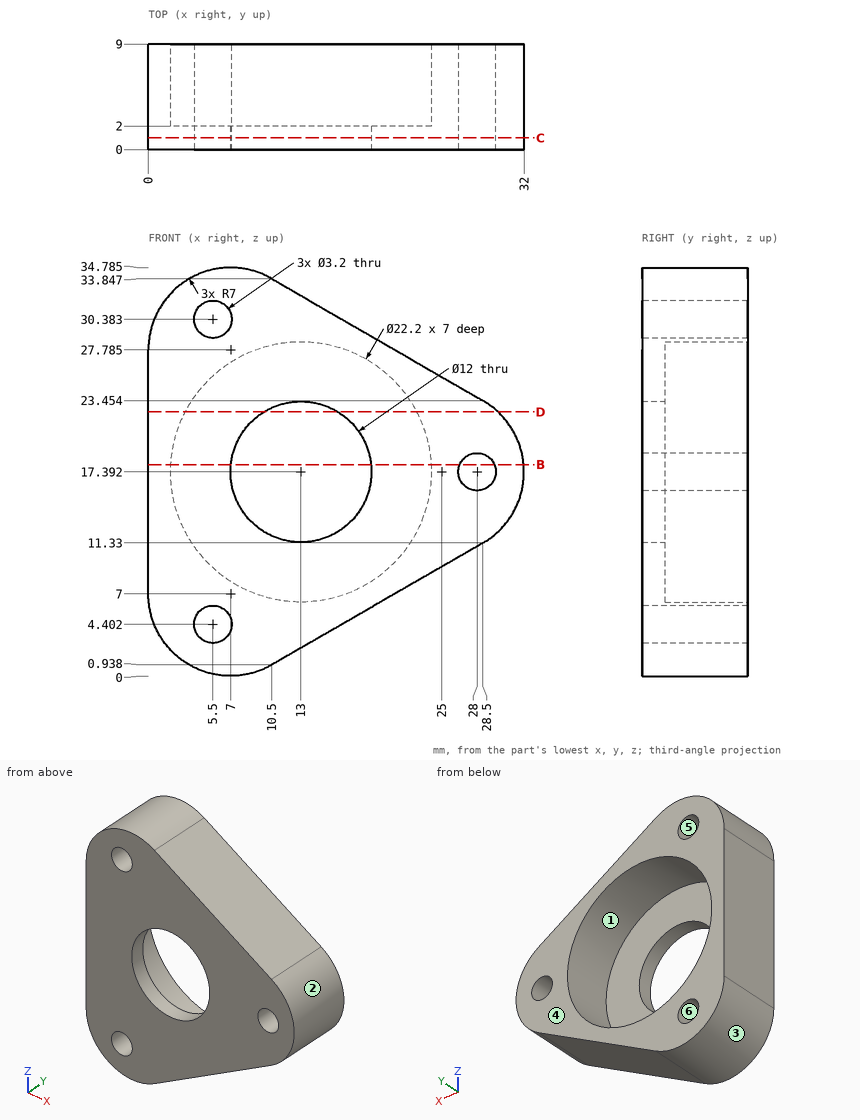
Here's the drawing with two shaded views (mm, measured from the low corner). I have some questions. A direction names the side the tool comes from. Coordinates: 2 decimals unless noted, no trailing zeros. Loops run counter-clockwise (first coordinate to the right, second up) from the corner with the lowest first, then second, coordinate; pieces in that order, holes last.
Item 1: Suppose I cut it at C-C (y = 1). Please give me the cut outline in (x, z) (1 decimal), then the cut area to 3 significant figures.
Answers below:
outline: (0, 7) arc R7 ccw to (10.5, 0.9) - (28.5, 11.3) arc R7 ccw to (28.5, 23.5) - (10.5, 33.8) arc R7 ccw to (0, 27.8) - close; hole circle Ø3.2 at (5.5, 4.4); hole circle Ø3.2 at (5.5, 30.4); hole circle Ø12 at (13, 17.4); hole circle Ø3.2 at (28, 17.4)
area: 640 mm2
Item 2: Which directions (+Z, -Z, +X, -X, +Y, -Y) give clear straight access to the entire face, cutting with the end or side of a thin tool? Please do the marked faces 1 and 2.
Answers below:
face 1: +Y
face 2: +X, +Y, -Y
Item 3: Suppose I cut it at B-B (z = 18). Please give me the cut outline in (x, y).
Answers below:
outline: (0, 0) - (7.03, 0) - (7.03, 2) - (1.92, 2) - (1.92, 9) - (0, 9) - close; (18.97, 0) - (26.52, 0) - (26.52, 9) - (24.08, 9) - (24.08, 2) - (18.97, 2) - close; (29.48, 0) - (31.97, 0) - (31.97, 9) - (29.48, 9) - close
Item 4: Suppose I cut it at D-D (z = 22.5). Please give me the cut outline in (x, y) (1 decimal).
Answers below:
outline: (0, 0) - (9.9, 0) - (9.9, 2) - (3.1, 2) - (3.1, 9) - (0, 9) - close; (16.1, 0) - (29.8, 0) - (29.8, 9) - (22.9, 9) - (22.9, 2) - (16.1, 2) - close
Item 5: I'm going to push flat-ended pins straight in: pin 1 (2 mm diameter, centred on y = 3, z = 15.5, fed in from +X); pin 2 (8 mm diameter, centred on x = 17.5, z = 15, fed in from +Y); pin 3 (5 mm diameter, centred on x = 10.5, y = 4, fed in from -Z). Where does each tip first touch, or does it pass through?
Answers below:
pin 1: stops at x = 31.94
pin 2: stops at y = 2
pin 3: stops at z = 0.07
Item 6: Please list where these lines run through material, in increasing order: L1, parallel to X at y = 1.25, z = 16 (1 decimal); L2, parallel to X at y = 6.75, z = 16 (1 decimal); L3, parallel to Z at x = 5.5, y = 2.5 (1 decimal).
Answers below:
L1: x = 0 to 7.2, 18.8 to 27.2, 28.8 to 31.9
L2: x = 0 to 2, 24 to 27.2, 28.8 to 31.9
L3: z = 0.2 to 2.8, 6 to 9.2, 25.6 to 28.8, 32 to 34.6
Item 7: If we mould it in two halves opening along Z, with no side actions, what happens to the marked faces 3, 4, 5 and 6? For each: released by +Z, released by -Z, zero draft, split by the parting line, or undercut.
Answers below:
face 3: released by -Z
face 4: zero draft
face 5: undercut
face 6: undercut
